from build123d import *

# Parameters (mm, degrees)
F0_W      = 35
F0_H      = 63
F1_DEPTH  = 35.3
F2_W      = 15
F2_H      = 2
F3_DEPTH  = 63.001
F4_DEPTH  = 63
F5_R      = 5
F6_DEPTH  = 23
F5_R_2    = 7.5
F7_DEPTH  = 5
F9_DEPTH  = 5
F11_DEPTH = 104
F13_DEPTH = 63
F14_R     = 5
F15_DEPTH = 23
F14_R_2   = 7.5
F16_DEPTH = 5
F17_R     = 1.75
F18_DEPTH = 5
F20_DEPTH = 5


with BuildPart() as f1:
    # F0 (on Top) → F1 (new body)
    with BuildSketch(Plane.XY):
        with Locations((-0.486111, -31.5)):
            Rectangle(F0_W, F0_H)
    extrude(amount=-F1_DEPTH)

    # F2 (on face) → F3 (cut, through all)
    with BuildSketch(Plane.XZ.offset(63)):
        with Locations((9.513889, -34.3)):
            Rectangle(F2_W, F2_H)
        with Locations((-10.486111, -34.3)):
            Rectangle(F2_W, F2_H)
    extrude(amount=-F3_DEPTH, mode=Mode.SUBTRACT)

    # F2 (on face) → F4 (join)
    with BuildSketch(Plane.XZ.offset(63)):
        Polygon((-17.986111, -19.1), (-17.986111, -12), (-24.006156, -15.55), align=None)
        Polygon((-17.986111, -26.2), (-17.986111, -19.1), (-24.006156, -22.65), align=None)
        Polygon((-17.986111, -33.3), (-17.986111, -26.2), (-24.006156, -29.75), align=None)
        Polygon((23.033934, -29.75), (17.013889, -26.2), (17.013889, -33.3), align=None)
        Polygon((23.033934, -15.55), (17.013889, -12), (17.013889, -19.1), align=None)
        Polygon((23.033934, -22.65), (17.013889, -19.1), (17.013889, -26.2), align=None)
    extrude(amount=-F4_DEPTH)

    # F5 (on face) → F6 (cut)
    with BuildSketch(Plane.XY):
        with Locations((-0.486111, -17)):
            Circle(F5_R)
        with Locations((-0.486111, -52)):
            Circle(F5_R)
    extrude(amount=-F6_DEPTH, mode=Mode.SUBTRACT)

    # F5 (on face) → F7 (cut)
    with BuildSketch(Plane.XY):
        with Locations((-0.486111, -17)):
            Circle(F5_R_2)
        with Locations((-0.486111, -17)):
            Circle(F5_R, mode=Mode.SUBTRACT)
        with Locations((-0.486111, -52)):
            Circle(F5_R_2)
        with Locations((-0.486111, -52)):
            Circle(F5_R, mode=Mode.SUBTRACT)
    extrude(amount=-F7_DEPTH, mode=Mode.SUBTRACT)

    # F8 (on face) → F9 (cut)
    with BuildSketch(Plane.XZ.offset(63)):
        Polygon((-0.486111, -25.3), (-7.986111, -25.3), (-7.986111, -35.504304), (7.013889, -35.504304), (7.013889, -25.3), align=None)
    extrude(amount=-F9_DEPTH, mode=Mode.SUBTRACT)

    # F10 (on face) → F11 (join)
    with BuildSketch(Plane(origin=(0, 0, 0), x_dir=(-1, 0, 0), z_dir=(0, 1, 0))):
        Polygon((17.986111, -2), (-17.013889, -2), (-17.013889, -12), (-23.033934, -15.55), (-17.013889, -19.1), (-23.033934, -22.65), (-17.013889, -26.2), (-23.033934, -29.75), (-17.013889, -33.3), (-2.013889, -33.3), (-2.013889, -35.3), (2.986111, -35.3), (2.986111, -33.3), (17.986111, -33.3), (24.006156, -29.75), (17.986111, -26.2), (24.006156, -22.65), (17.986111, -19.1), (24.006156, -15.55), (17.986111, -12), align=None)
    extrude(amount=F11_DEPTH)

    # F12 (on face) → F13 (join)
    with BuildSketch(Plane(origin=(0, 104, 0), x_dir=(-1, 0, 0), z_dir=(0, 1, 0))):
        Polygon((17.986111, 0), (-17.013889, 0), (-17.013889, -12), (-23.033934, -15.55), (-17.013889, -19.1), (-23.033934, -22.65), (-17.013889, -26.2), (-23.033934, -29.75), (-17.013889, -33.3), (-2.013889, -33.3), (-2.013889, -35.3), (2.986111, -35.3), (2.986111, -33.3), (17.986111, -33.3), (24.006156, -29.75), (17.986111, -26.2), (24.006156, -22.65), (17.986111, -19.1), (24.006156, -15.55), (17.986111, -12), align=None)
    extrude(amount=F13_DEPTH)

    # F14 (on face) → F15 (cut)
    with BuildSketch(Plane.XY):
        with Locations((-0.486111, 156)):
            Circle(F14_R)
        with Locations((-0.486111, 121)):
            Circle(F14_R)
    extrude(amount=-F15_DEPTH, mode=Mode.SUBTRACT)

    # F14 (on face) → F16 (cut)
    with BuildSketch(Plane.XY):
        with Locations((-0.486111, 156)):
            Circle(F14_R_2)
        with Locations((-0.486111, 156)):
            Circle(F14_R, mode=Mode.SUBTRACT)
        with Locations((-0.486111, 121)):
            Circle(F14_R_2)
        with Locations((-0.486111, 121)):
            Circle(F14_R, mode=Mode.SUBTRACT)
    extrude(amount=-F16_DEPTH, mode=Mode.SUBTRACT)

    # F17 (on face) → F18 (join)
    with BuildSketch(Plane(origin=(0, 0, -35.3), x_dir=(1, 0, 0), z_dir=(0, 0, -1))):
        with Locations((-0.486111, -52)):
            Circle(F17_R)
    extrude(amount=F18_DEPTH)

    # F19 (on face) → F20 (cut)
    with BuildSketch(Plane(origin=(0, 167, 0), x_dir=(-1, 0, 0), z_dir=(0, 1, 0))):
        Polygon((7.986111, -25.3), (0.486111, -25.3), (-7.013889, -25.3), (-7.013889, -35.3), (0.486111, -35.3), (7.986111, -35.3), align=None)
    extrude(amount=-F20_DEPTH, mode=Mode.SUBTRACT)


solid = f1.part
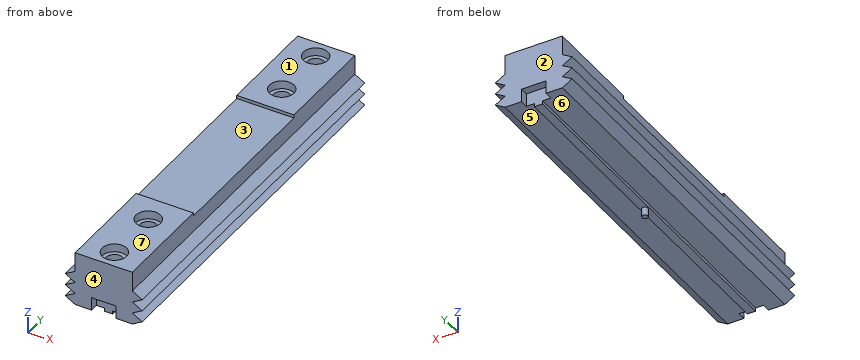
Can you work these out from the model? Positions are in its coordinate system, mm. Face numbers are marked on the shaded views. A direction names the side the tool comes from. Give positions to 0.01 mm unless a question says otherwise; leave off trailing zeros. Order: outer loops, then holes, each group sorted by start corner. A loop starts at its lowest first (then second) coordinate and runs counter-clockwise, first axis right, second up. Notation, with made-up numbers: M -11.75,58.5 L 19.25,58.5 A14 cw 19.25,66.5 Z; hole C 28.25,-37 d1. An arc over 180 degrees is marked long. One line per item, written item: value.
Item 1: If we section it at B-B on x = -15: Write out the boundary of the cut face in (y, z), and give its area (3 significant figures).
Verdict:
outline: M -63,-33.3 L 167,-33.3 L 167,0 L 104,0 L 104,-2 L 0,-2 L 0,0 L -63,0 Z
area: 7,450 mm2
Item 2: For pin 1 (2.5 mm diameter, centred on x = -1.5, y = 17, fed in from -Z); pin 2 (1.5 mm diameter, centred on y = 165.5, z = -29.5, fed in from +X); pin 3 (1 mm diameter, centred on y = 95.5, z = -34, fed in from +X), each with a flat end and sliding along its axis, tell me the tip position at first contact or that it passes through.
Verdict:
pin 1: z = -35.3
pin 2: x = 23.03
pin 3: x = 2.01
Item 3: For the marked faces 5, 6 and 7, which set-ups out of +Z, -Z, +X, -X, +Y, -Y let a thin tool reach every point of the face, with its end or its side?
Verdict:
face 5: -Z, +X, +Y, -Y
face 6: -Z, -X, +Y, -Y
face 7: +Z, +X, -X, +Y, -Y
Item 4: If we mould it in two halves opening along Y, with no side actions, what happens to the marked faces 1, 2, 3 and 4? For each: pulls with the +Y half, pulls with the -Y half, needs draft (parallel to the pull), parting line crosses it, or undercut.
Verdict:
face 1: needs draft
face 2: pulls with the +Y half
face 3: undercut
face 4: pulls with the -Y half
Item 5: Please list where these lines run through material, in increasing order: line 1 (Y direction, x = -5, z = -16.5); line 2 (Z direction, x = -16.5, y = 90); line 3 (Z direction, x = -14.5, y = -38.5).
Verdict:
line 1: -63 to -54.15, -49.85 to -19.15, -14.85 to 118.85, 123.15 to 153.85, 158.15 to 167
line 2: -33.3 to -2
line 3: -33.3 to 0
Item 6: If we section it at A-A on y = 121: Write out the boundary of the cut face in (x, z).
Verdict:
outline: M -24.01,-29.75 L -17.99,-33.3 L -2.99,-33.3 L -2.99,-35.3 L 2.01,-35.3 L 2.01,-33.3 L 17.01,-33.3 L 23.03,-29.75 L 17.01,-26.2 L 23.03,-22.65 L 17.01,-19.1 L 23.03,-15.55 L 17.01,-12 L 17.01,0 L 7.01,0 L 7.01,-5 L 4.51,-5 L 4.51,-23 L -5.49,-23 L -5.49,-5 L -7.99,-5 L -7.99,0 L -17.99,0 L -17.99,-12 L -24.01,-15.55 L -17.99,-19.1 L -24.01,-22.65 L -17.99,-26.2 Z
